Job drawing, mm, ordinate dimensions from the low corner. One solid piece. A direction names the side the tool comes from. Give positions to 0.01 mm unless a question says otherwise; leave off trailing zeros. Write each loop counter-clockwise with the first axis right and the second up, starting at its lowest first coordinate (ties: lowest second). Pieces come first, ordered by that corner, then holes. Notation, with made-up numbers: (55.5, 24) - (109.5, 24) arc R16 ccw to (109.5, 38) - close; hole circle Ø3 at (31, -25). An arc over 180 degrees is marked (long way). Answer in a Markdown table with one row per item. Add a question column.
1. Drop flat-ended pins along their axis: pin 1 Ø10 at (x, y) = (38.1, 12.7) entering from -Z; pin 2 Ø20.5 at (x, z) = (63.5, 19.05) entering from -Y; pin 3 Ø12 at (y, z) = (36, 107.5) entering from -X; pin 4 Ø12 at (x, y) = (51, 10) entering from +Z. Give the stop position or say it passes through.
2. Probe line 1 along Z through (x, y) = (63.5, 81); line 2 along Y through (x, z) = (38.1, 105.25); line 3 along Z through (x, y) = (41, 20). List the from-to ranges inside material, lowest first.
3. Pull direction Z, two halves, no side cores. Call the marked faces 4, 5, 6 and 7: released by +Z, released by -Z, zero draft, split by the parting line, or undercut.
4. Band-saw the part on A-A on z = 19.05. Write the cut outline in (x, y).
5. Band-saw the part on B-B on y = 23. Write the cut outline in (x, z), plus the area to 3 significant figures.
6. Band-saw the part on C-C on x = 63. Write the cut outline in (y, z).
7. Which spindle directions (+Z, -Z, +X, -X, +Y, -Y) get a long thin tool onto all of the face, cutting with end or side? Do the marked faces 1, 2 and 3. Say none if no direction does.
8. Band-saw the part on D-D on y = 11. Write the cut outline in (x, z).
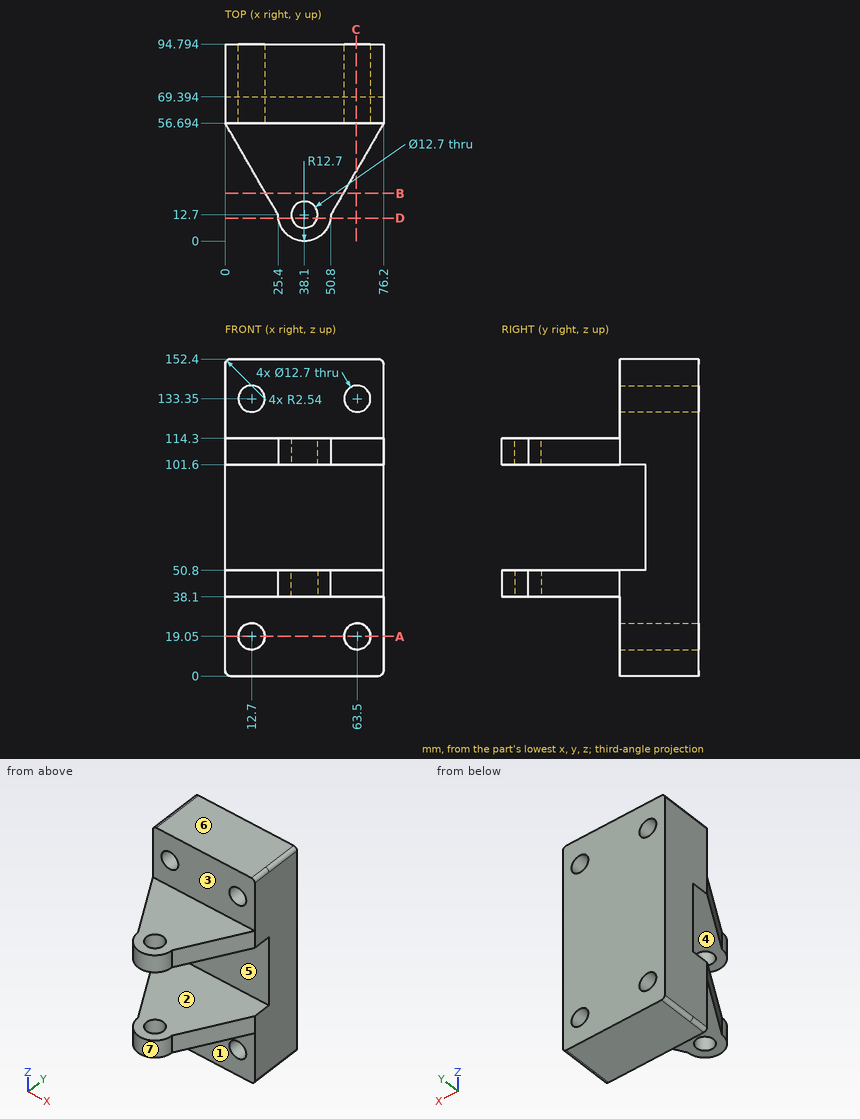
Values:
| question | item | result |
|---|---|---|
| 1 | pin 1 | passes through |
| 1 | pin 2 | stops at y = 56.69 |
| 1 | pin 3 | stops at x = 8.48 |
| 1 | pin 4 | stops at z = 114.3 |
| 2 | line 1 | z = 0 to 12.7, 25.4 to 127, 139.7 to 152.4 |
| 2 | line 2 | y = 0 to 6.35, 19.05 to 94.79 |
| 2 | line 3 | z = 38.1 to 50.8, 101.6 to 114.3 |
| 3 | face 4 | undercut |
| 3 | face 5 | undercut |
| 3 | face 6 | released by +Z |
| 3 | face 7 | zero draft |
| 4 | outline | (0, 56.69) - (6.35, 56.69) - (6.35, 94.79) - (0, 94.79) - close; (19.05, 56.69) - (57.15, 56.69) - (57.15, 94.79) - (19.05, 94.79) - close; (69.85, 56.69) - (76.2, 56.69) - (76.2, 94.79) - (69.85, 94.79) - close |
| 5 | outline | (19.45, 38.1) - (56.75, 38.1) - (56.75, 50.8) - (19.45, 50.8) - close; (19.45, 101.6) - (56.75, 101.6) - (56.75, 114.3) - (19.45, 114.3) - close |
| 5 | area | 947 mm² |
| 6 | outline | (33.83, 38.1) - (56.69, 38.1) - (56.69, 25.38) - (94.79, 25.38) - (94.79, 127.02) - (56.69, 127.02) - (56.69, 114.3) - (33.83, 114.3) - (33.83, 101.6) - (69.39, 101.6) - (69.39, 50.8) - (33.83, 50.8) - close; (56.69, 0) - (94.79, 0) - (94.79, 12.72) - (56.69, 12.72) - close; (56.69, 139.68) - (94.79, 139.68) - (94.79, 152.4) - (56.69, 152.4) - close |
| 7 | face 1 | -Z, +X, -X, -Y |
| 7 | face 2 | +X, -X, -Y |
| 7 | face 3 | +Z, +X, -X, -Y |
| 8 | outline | (25.51, 38.1) - (31.98, 38.1) - (31.98, 50.8) - (25.51, 50.8) - close; (25.51, 101.6) - (31.98, 101.6) - (31.98, 114.3) - (25.51, 114.3) - close; (44.22, 38.1) - (50.69, 38.1) - (50.69, 50.8) - (44.22, 50.8) - close; (44.22, 101.6) - (50.69, 101.6) - (50.69, 114.3) - (44.22, 114.3) - close |
